from build123d import *

# Parameters (mm, degrees)
SKETCH1_W               = 114.3
SKETCH1_H               = 21.59
SKETCH1_R               = 4.191
BOSS_EXTRUDE1_DEPTH     = 6.35
SKETCH2_W               = 9.525
SKETCH2_H               = 6.35
BOSS_EXTRUDE2_DEPTH     = 17.4625
SKETCH3_W               = 9.525
SKETCH3_H               = 6.35
BOSS_EXTRUDE3_DEPTH     = 17.4625
SKETCH4_W               = 9.525
SKETCH4_H               = 6.35
BOSS_EXTRUDE4_DEPTH     = 17.78
SKETCH6_W               = 9.525
SKETCH6_H               = 9.525
BOSS_EXTRUDE5_DEPTH     = 12.7
CUT_EXTRUDE1_DEPTH      = 53.848
CUT_EXTRUDE1_DEPTH_BACK = 92.456
SKETCH7_R               = 2.667
BOSS_EXTRUDE6_DEPTH     = 6.35
CUT_EXTRUDE2_START      = -6.35
SKETCH10_R              = 4.191
CUT_EXTRUDE2_DEPTH      = 6.35
SKETCH11_R              = 7.14375
CUT_EXTRUDE3_DEPTH      = 6.73125


with BuildPart() as part:
    # Sketch1 → Boss-Extrude1 (new body)
    with BuildSketch(Plane(origin=(0, 0, 0), x_dir=(1, 0, 0), z_dir=(0, 1, 0))):
        Rectangle(SKETCH1_W, SKETCH1_H)
        with Locations(Location((0, 0, 0), (0, 0, 270))):
            Circle(SKETCH1_R, mode=Mode.SUBTRACT)
    extrude(amount=BOSS_EXTRUDE1_DEPTH)

    # Sketch2 → Boss-Extrude2 (add)
    with BuildSketch(Plane(origin=(0, 0, -10.795), x_dir=(-1, 0, 0), z_dir=(0, 0, -1))):
        with Locations((-52.3875, 3.175)):
            Rectangle(SKETCH2_W, SKETCH2_H)
    extrude(amount=BOSS_EXTRUDE2_DEPTH)

    # Sketch3 → Boss-Extrude3 (add)
    with BuildSketch(Plane(origin=(0, 0, -10.795), x_dir=(-1, 0, 0), z_dir=(0, 0, -1))):
        with Locations((52.3875, 3.175)):
            Rectangle(SKETCH3_W, SKETCH3_H)
    extrude(amount=BOSS_EXTRUDE3_DEPTH)

    # Sketch4 → Boss-Extrude4 (add)
    with BuildSketch(Plane.XY.offset(10.795)):
        with Locations((-52.3875, 3.175)):
            Rectangle(SKETCH4_W, SKETCH4_H)
        with Locations((52.3875, 3.175)):
            Rectangle(SKETCH4_W, SKETCH4_H)
    extrude(amount=BOSS_EXTRUDE4_DEPTH)

    # Sketch6 → Boss-Extrude5 (add)
    with BuildSketch(Plane(origin=(0, 6.35, 0), x_dir=(1, 0, 0), z_dir=(0, 1, 0))):
        with Locations((-52.3875, 23.495)):
            Rectangle(SKETCH6_W, SKETCH6_H)
        with Locations((-52.3875, -23.8125)):
            Rectangle(SKETCH6_W, SKETCH6_H)
        with Locations((52.3875, 23.495)):
            Rectangle(SKETCH6_W, SKETCH6_H)
        with Locations((52.3875, -23.8125)):
            Rectangle(SKETCH6_W, SKETCH6_H)
    extrude(amount=BOSS_EXTRUDE5_DEPTH)

    # Sketch7 → Cut-Extrude1 (cut, two sides: drawn at the far end of the back side and taken through both)
    with BuildSketch(Plane(origin=(0, 0, -28.2575), x_dir=(-1, 0, 0), z_dir=(0, 0, -1)).offset(-CUT_EXTRUDE1_DEPTH_BACK)):
        with Locations(Location((-52.3875, 12.7, 0), (0, 0, 180))):
            Circle(SKETCH7_R)
        with Locations(Location((52.3875, 12.7, 0), (0, 0, 180))):
            Circle(SKETCH7_R)
    extrude(amount=CUT_EXTRUDE1_DEPTH + CUT_EXTRUDE1_DEPTH_BACK, mode=Mode.SUBTRACT)

    # Sketch9 → Boss-Extrude6 (add)
    with BuildSketch(Plane.XZ):
        Polygon((57.15, -28.2575), (57.15, 28.575), (47.625, 28.575), (47.625, 10.795), (-47.625, 10.795), (-47.625, 28.575), (-57.15, 28.575), (-57.15, -28.2575), (-47.625, -28.2575), (-47.625, -10.795), (47.625, -10.795), (47.625, -28.2575), align=None)
    extrude(amount=BOSS_EXTRUDE6_DEPTH)

    # Sketch10 → Cut-Extrude2 (cut)
    with BuildSketch(Plane(origin=(0, 0, 0), x_dir=(1, 0, 0), z_dir=(0, 1, 0)).offset(CUT_EXTRUDE2_START)):
        with Locations(Location((0, 0, 0), (0, 0, 90))):
            Circle(SKETCH10_R)
    extrude(amount=CUT_EXTRUDE2_DEPTH, mode=Mode.SUBTRACT)

    # Sketch11 → Cut-Extrude3 (cut)
    with BuildSketch(Plane.XZ.offset(6.35)):
        with Locations(Location((0, 0, 0), (0, 0, 270))):
            Circle(SKETCH11_R)
    extrude(amount=-CUT_EXTRUDE3_DEPTH, mode=Mode.SUBTRACT)


solid = part.part
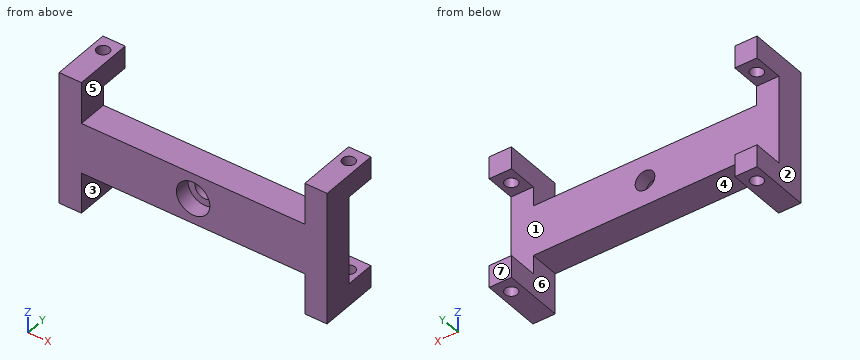
Can you work these out from the model? Positions are in its coordinate system, mm. Face numbers are marked on the shaded views. A direction names the side the tool comes from. Coordinates: 2 decimals unless noted, no trailing zeros. Write each loop counter-clockwise with the first axis right and the second up, starting at its lowest first coordinate (ties: lowest second). Pieces come first, ordered by that corner, then holes. Notation, with made-up numbers: (22.25, -4) -> (48.25, -4) arc R16 ccw to (48.25, 21) -> close; hole circle Ø1 at (24, -19). An arc over 180 degrees is marked (long way). Write each question's results on one line, items separated by ' | '. Start each with the question number.
Item 1: On a 3-axis mill with a long thin cutter (end or side, diameter ignored), from which of +Z, -Z, +X, -X, +Y, -Y can I reach the whole of each face in a straight line? I mean the marked faces 5, 6 and 7. Say none if no direction works.
Item 2: If we section it at A-A, the plane x = 0: Write out the boundary of the cut face in (y, z) (3 decimals).
Item 3: If we section it at C-C, the plane z = 0: Write out the boundary of the cut face in (x, y), and give its area (3 significant figures).
Item 4: If we section it at B-B, the plane y = 12.7: Count the separate pieces of the cut face and the enclosed holes in it, and give its area (3 significant figures).
Item 5: Please list where these lines run through material, in increasing order: probe 1 along Z at (x, y) = (0, 3.15) (3 decimals); probe 2 along X at (y, z) = (3.05, 0); probe 3 along X at (y, z) = (8.5, 20.5) (3 decimals).
Item 6: I'm going to push flat-ended pins straight in: P1, Ø5, axis at x = -52.39, y = 12.7, coming from the -Z side; P2, Ø8.5, axis at x = 0, z = 0, coming from the +Y side; P3, Ø14, axis at x = 12, y = -0.5, coming from the -Z side (3 decimals); P4, Ø9.5, axis at x = 0, z = 0, coming from the -Y side. Where does each tip first touch, or does it pass through?
Item 7: Thinking about a two-plate mould opening in X: for the marked faces 1, 2, 3 and 4, which applies, released by +X, released by -X, zero draft, split by the parting line, or undercut?
Answer block:
1) face 5: +Z, +Y, -Y | face 6: -Z, +Y, -Y | face 7: +Z, -Z, +X, -X, +Y
2) outline: (-6.35, -10.795) -> (6.35, -10.795) -> (6.35, -4.191) -> (0.381, -4.191) -> (0.381, -7.144) -> (-6.35, -7.144) -> close; (-6.35, 7.144) -> (0.381, 7.144) -> (0.381, 4.191) -> (6.35, 4.191) -> (6.35, 10.795) -> (-6.35, 10.795) -> close
3) outline: (-57.15, -6.35) -> (-7.14, -6.35) -> (-7.14, 0.38) -> (-4.19, 0.38) -> (-4.19, 6.35) -> (-57.15, 6.35) -> close; (4.19, 0.38) -> (7.14, 0.38) -> (7.14, -6.35) -> (57.15, -6.35) -> (57.15, 6.35) -> (4.19, 6.35) -> close | area: 1,310 mm²
4) separate pieces: 8 | enclosed holes: 0 | area: 160 mm²
5) probe 1: -10.795 to -4.191, 4.191 to 10.795 | probe 2: -57.15 to -4.19, 4.19 to 57.15 | probe 3: -57.15 to -47.625, 47.625 to 57.15
6) P1: through | P2: y = 6.35 | P3: z = -10.795 | P4: y = 0.38
7) face 1: zero draft | face 2: released by -X | face 3: undercut | face 4: undercut
